```python
from build123d import *

# Parameters (mm, degrees)
BOSS_EXTRUDE1_DEPTH                            = 12.7
SKETCH2_R                                      = 3.302
CUT_EXTRUDE1_DEPTH                             = 12.7
CBORE_FOR_4_SOCKET_HEAD_CAP_SCREW1_D           = 3.2639
CBORE_FOR_4_SOCKET_HEAD_CAP_SCREW1_CBORE_D     = 5.08
CBORE_FOR_4_SOCKET_HEAD_CAP_SCREW1_CBORE_DEPTH = 2.8448
SKETCH9_R                                      = 1.3462
CUT_EXTRUDE3_DEPTH                             = 8.89


with BuildPart() as part:
    # Sketch1 → Boss-Extrude1 (new body)
    with BuildSketch(Plane.XY):
        with BuildLine():
            Line((-12.7, 0), (-12.7, 13.208))
            Line((-12.7, 13.208), (12.7, 13.208))
            Line((12.7, 13.208), (12.7, 0))
            ThreePointArc((12.7, 0), (0, -12.7), (-12.7, 0))
        make_face()
    extrude(amount=BOSS_EXTRUDE1_DEPTH)

    # Sketch2 → Cut-Extrude1 (cut)
    with BuildSketch(Plane.XY.offset(12.7)):
        Circle(SKETCH2_R)
    extrude(amount=-CUT_EXTRUDE1_DEPTH, mode=Mode.SUBTRACT)

    # CBORE for #4 Socket Head Cap Screw1 (through all)
    with Locations(Plane.XY.offset(12.7)):
        with Locations((-9.525, 0), (0, 9.525), (9.525, 0), (0, -9.525)):
            CounterBoreHole(CBORE_FOR_4_SOCKET_HEAD_CAP_SCREW1_D / 2, CBORE_FOR_4_SOCKET_HEAD_CAP_SCREW1_CBORE_D / 2, CBORE_FOR_4_SOCKET_HEAD_CAP_SCREW1_CBORE_DEPTH)

    # Sketch9 → Cut-Extrude3 (cut)
    with BuildSketch(Plane(origin=(0, 13.208, 0), x_dir=(1, 0, 0), z_dir=(0, 1, 0))):
        with Locations((-7.62, -6.35)):
            Circle(SKETCH9_R)
        with Locations((7.62, -6.35)):
            Circle(SKETCH9_R)
    extrude(amount=-CUT_EXTRUDE3_DEPTH, mode=Mode.SUBTRACT)


solid = part.part
```
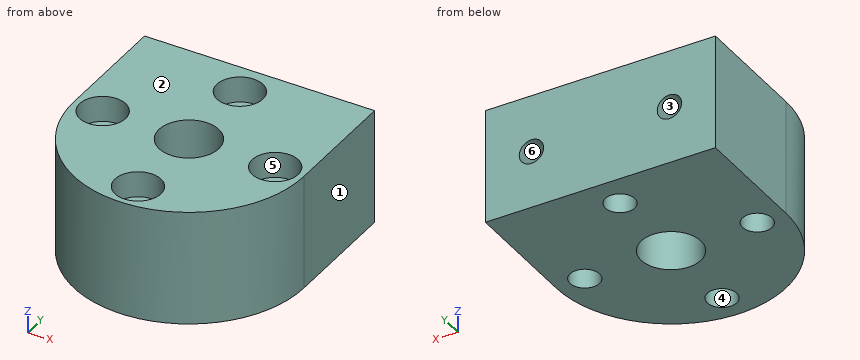
Here's how the part is built. I have some questions about the finished solid (model axes, mm). Face numbers are marked on the shaded views. A direction names the side the tool comes from. Coordinates: 2 decimals unless noted, no trailing zeros. Write each loop counter-clockwise with the first axis right and the second up, starting at its lowest first coordinate (ties: lowest second). Pieces come first, ordered by that corner, then holes. Notation, with made-up numbers: M 62.5,81 L 74.5,81 A13 ccw 74.5,96 Z; hole C 63,6.5 d5. An arc over 180 degrees is marked long. Answer as CSV lines item,"result". Start each with the question number.
Q1. I need wall thicknesses on probe 1 along Y at (x, z) = (0, 11.35) (3 decimals); probe 2 along Y at (x, z) = (-1.25, 6.25); probe 3 along X at (y, z) = (9.5, 7.75). Which ranges of each line are inside material? Lowest first, please. Write a range as [from, to].
Q2. Suppose I cut it at C-C, the plane z = 6. List the corners of the cut face in (x, y) for me (3 decimals), then the cut area to 3 significant figures.
Q3. Suppose I cut it at D-D, the plane x = -10.75. List the corners of the cut face in (y, z) for me.
Q4. Suppose I cut it at A-A, the plane x = 0. List the corners of the cut face in (y, z) for me (3 decimals), then the cut area to 3 significant figures.
Q5. Suppose I cut it at B-B, the plane y = 5. List the corners of the cut face in (x, z) for me, then the cut area to 3 significant figures.
Q6. If we mould it in two halves opening along X, with no side actions, what happens to the marked faces 1, 2 and 3? For each: pulls with the +X half, pulls with the -X half, needs draft (parallel to the pull), parting line crosses it, or undercut.
Q7. For the marked faces 4, 5 and 6, which set-ups out of +Z, -Z, +X, -X, +Y, -Y let a thin tool reach every point of the face, with its end or its side?
Q8. Will these pins go through, and if not, where does the flat tip stop? pin 1 Ø1.5 at (y, z) = (-2.5, 10) entering from +X; pin 2 Ø1 at (x, z) = (-4.5, 2) entering from -Y; pin 3 Ø4 at (y, z) = (-5, 5.5) entering from -X.
Entries:
1,probe 1,"y = [-12.7, -12.065], [-6.985, -3.302], [3.302, 6.985], [12.065, 13.208]"
1,probe 2,"y = [-12.64, -10.57], [-8.48, -3.06], [3.06, 8.48], [10.57, 13.21]"
1,probe 3,"x = [-12.7, -1.63], [1.63, 12.7]"
2,outline,"M -12.7,0 A12.7 ccw 12.7,0 L 12.7,13.208 L 8.92,13.208 L 8.92,4.318 L 6.32,4.318 L 6.32,13.208 L -6.32,13.208 L -6.32,4.318 L -8.92,4.318 L -8.92,13.208 L -12.7,13.208 Z; hole C -9.525,0 d3.264; hole C 0,0 d6.604; hole C 0,-9.525 d3.264; hole C 0,9.525 d3.264; hole C 9.525,0 d3.264"
2,area,"475 mm²"
3,outline,"M -6.76,0 L -1.08,0 L -1.08,9.86 L -2.23,9.86 L -2.23,12.7 L -6.76,12.7 Z; M 1.08,0 L 13.21,0 L 13.21,12.7 L 2.23,12.7 L 2.23,9.86 L 1.08,9.86 Z"
4,outline,"M -12.7,0 L -11.157,0 L -11.157,9.855 L -12.065,9.855 L -12.065,12.7 L -12.7,12.7 Z; M -7.893,0 L -3.302,0 L -3.302,12.7 L -6.985,12.7 L -6.985,9.855 L -7.893,9.855 Z; M 3.302,0 L 7.893,0 L 7.893,9.855 L 6.985,9.855 L 6.985,12.7 L 3.302,12.7 Z; M 11.157,0 L 13.208,0 L 13.208,12.7 L 12.065,12.7 L 12.065,9.855 L 11.157,9.855 Z"
4,area,"152 mm²"
5,outline,"M -12.7,0 L 12.7,0 L 12.7,12.7 L -12.7,12.7 Z; hole C -7.62,6.35 d2.69; hole C 7.62,6.35 d2.69"
5,area,"311 mm²"
6,face 1,"pulls with the +X half"
6,face 2,"needs draft"
6,face 3,"undercut"
7,face 4,"+Z, -Z"
7,face 5,"+Z"
7,face 6,"+Y"
8,pin 1,"stops at x = 12.58"
8,pin 2,"stops at y = -12.05"
8,pin 3,"stops at x = -12.34"
